from build123d import *

# Parameters (mm, degrees)
SKETCH1_W               = 167
SKETCH1_H               = 140.66
BOSS_EXTRUDE1_DEPTH     = 2
BOSS_EXTRUDE1_DRAFT     = -45
CUT_EXTRUDE1_REACH      = 220.353
SKETCH2_W               = 167
SKETCH2_H               = 140.66
SKETCH2_W_2             = 165
SKETCH2_H_2             = 138.66
BOSS_EXTRUDE2_START     = 120
BOSS_EXTRUDE2_DEPTH     = 22
CUT_EXTRUDE2_REACH      = 211.584
SKETCH4_W               = 20
SKETCH4_H               = 20
CUT_EXTRUDE3_DEPTH      = 218.119588246
CUT_EXTRUDE3_DEPTH_BACK = 218.119588246
SKETCH5_W               = 9
SKETCH5_H               = 9
CUT_EXTRUDE4_REACH      = 219.12
SKETCH6_W               = 59.5
SKETCH6_H               = 89
SKETCH7_W               = 35
SKETCH7_H               = 51
CUT_EXTRUDE5_DEPTH      = 2
BOSS_EXTRUDE4_START     = -2
SKETCH11_W              = 39
SKETCH11_H              = 55
BOSS_EXTRUDE4_DEPTH     = 1
CUT_EXTRUDE6_DEPTH      = 218.119588246
CUT_EXTRUDE6_DEPTH_BACK = 218.119588246
SKETCH12_W              = 9
SKETCH12_H              = 9


with BuildPart() as part:
    # Sketch1 → Boss-Extrude1 (with draft: the straight prism first)
    with BuildSketch(Plane(origin=(0, 0, 0), x_dir=(1, 0, 0), z_dir=(0, 1, 0))):
        with Locations((83.5, 70.33)):
            Rectangle(SKETCH1_W, SKETCH1_H)
    extrude(amount=-BOSS_EXTRUDE1_DEPTH)
    # Boss-Extrude1: the draft: its side faces are tilted about the plane it starts from
    boss_extrude1_sides = [part.faces().sort_by_distance(p)[0] for p in [
        (83.5, -1, 0),
        (167, -1, -70.33),
        (83.5, -1, -140.66),
        (0, -1, -70.33),
    ]]
    draft(boss_extrude1_sides, Plane(origin=(0, 0, 0), x_dir=(1, 0, 0), z_dir=(0, 1, 0)), BOSS_EXTRUDE1_DRAFT)

    # Sketch2 → Cut-Extrude1 (cut, up to next)
    with BuildSketch(Plane.XZ.offset(2), mode=Mode.PRIVATE) as cut_extrude1_sk1:
        with Locations((83.5, -70.33)):
            Rectangle(SKETCH2_W, SKETCH2_H)
        with Locations((83.5, -70.33)):
            Rectangle(SKETCH2_W_2, SKETCH2_H_2, mode=Mode.SUBTRACT)
    cut_extrude1_tool1 = extrude(cut_extrude1_sk1.sketch, amount=-CUT_EXTRUDE1_REACH, mode=Mode.PRIVATE) & part.part
    add(cut_extrude1_tool1.solids().sort_by_distance((83.5, -2, -140.441656))[0], mode=Mode.SUBTRACT)

    # Sketch3 → Boss-Extrude2 (add)
    with BuildSketch(Plane(origin=(0, 0, 0), x_dir=(0, 0, -1), z_dir=(1, 0, 0)).offset(BOSS_EXTRUDE2_START)):
        Polygon((76.33, 0), (84.33, 8.94427191), (103.33, 0), align=None)
    extrude(amount=BOSS_EXTRUDE2_DEPTH)

    # Cut-Extrude2: up to this plane
    cut_extrude2_end = Plane(origin=(0, -2, 0), z_dir=(0, -1, 0))
    # Sketch4 → Cut-Extrude2 (cut, up to the surface)
    with BuildSketch(Plane(origin=(0, 39.818641072, -18.744671202), x_dir=(1, 0, 0), z_dir=(0, 0.9047619047619048, -0.42591770999996015)), mode=Mode.PRIVATE) as cut_extrude2_sk1:
        with Locations((131, 83.489047619)):
            Rectangle(SKETCH4_W, SKETCH4_H)
    cut_extrude2_tool1 = split(extrude(cut_extrude2_sk1.sketch, amount=-CUT_EXTRUDE2_REACH, mode=Mode.PRIVATE), bisect_by=cut_extrude2_end, keep=Keep.BOTH, mode=Mode.PRIVATE)
    add(cut_extrude2_tool1.solids().sort_by_distance((131, 4.259177, -94.282381))[0], mode=Mode.SUBTRACT)

    # Sketch5 → Cut-Extrude3 (cut, two sides: drawn at the far end of the back side and taken through both)
    with BuildSketch(Plane(origin=(0, 0, 0), x_dir=(1, 0, 0), z_dir=(0, 1, 0)).offset(-CUT_EXTRUDE3_DEPTH_BACK)):
        with Locations((92, 90.33)):
            Rectangle(SKETCH5_W, SKETCH5_H)
        with Locations((92, 52.33)):
            Rectangle(SKETCH5_W, SKETCH5_H)
        with Locations((70, 52.33)):
            Rectangle(SKETCH5_W, SKETCH5_H)
    extrude(amount=CUT_EXTRUDE3_DEPTH + CUT_EXTRUDE3_DEPTH_BACK, mode=Mode.SUBTRACT)

    # Sketch6 → Cut-Extrude4 (cut, up to next)
    with BuildSketch(Plane(origin=(0, 0, 0), x_dir=(1, 0, 0), z_dir=(0, 1, 0)), mode=Mode.PRIVATE) as cut_extrude4_sk1:
        with Locations((31.75, 79.33)):
            Rectangle(SKETCH6_W, SKETCH6_H)
    cut_extrude4_tool1 = extrude(cut_extrude4_sk1.sketch, amount=-CUT_EXTRUDE4_REACH, mode=Mode.PRIVATE) & part.part
    add(cut_extrude4_tool1.solids().sort_by_distance((31.75, 0, -79.33))[0], mode=Mode.SUBTRACT)

    # Sketch7 → Cut-Extrude5 (cut)
    with BuildSketch(Plane(origin=(0, 0, 0), x_dir=(1, 0, 0), z_dir=(0, 1, 0))):
        with Locations((81, 71.33)):
            Rectangle(SKETCH7_W, SKETCH7_H)
    extrude(amount=-CUT_EXTRUDE5_DEPTH, mode=Mode.SUBTRACT)

    # Sketch11 → Boss-Extrude4 (add)
    with BuildSketch(Plane(origin=(0, 0, 0), x_dir=(1, 0, 0), z_dir=(0, 1, 0)).offset(BOSS_EXTRUDE4_START)):
        with Locations((81, 71.33)):
            Rectangle(SKETCH11_W, SKETCH11_H)
    extrude(amount=-BOSS_EXTRUDE4_DEPTH)

    # Sketch12 → Cut-Extrude6 (cut, two sides: drawn at the far end of the back side and taken through both)
    with BuildSketch(Plane(origin=(0, 0, 0), x_dir=(1, 0, 0), z_dir=(0, 1, 0)).offset(-CUT_EXTRUDE6_DEPTH_BACK)):
        with Locations((92, 52.33)):
            Rectangle(SKETCH12_W, SKETCH12_H)
        with Locations((70, 52.33)):
            Rectangle(SKETCH12_W, SKETCH12_H)
        with Locations((92, 90.33)):
            Rectangle(SKETCH12_W, SKETCH12_H)
    extrude(amount=CUT_EXTRUDE6_DEPTH + CUT_EXTRUDE6_DEPTH_BACK, mode=Mode.SUBTRACT)


solid = part.part
Design review of the part built by this model. Coordinates are the model's own, in mm. A direction names the side the tool comes from. Coordinates: 2 decimals unless noted, no trailing zeros. Order: outer loops, then holes, each group sorted by start corner. A loop starts at its lowest first (then second) coordinate and runs counter-clockwise, first axis right, second up. Notation, with made-up numbers: (37, 47.5) -> (81, 47.5) arc R3 ccw to (81, 51.5) -> close; hole circle Ø2 at (77.25, 22.25). An arc over 180 degrees is marked (long way). Use one line per item in the form item = value. Start each with the question number.
(1) Add section C-C on z = -64. State the section outline as (x, y) points.
(2) Add section B-B on x = 47. State the section outline as (y, z) points.
(3) For faces 5 (the flat face through (81, -2, -72)), 6 (the flat face through (130.95, 8.8, -84.64)), list the 3-axis set-ups (+Z, -Z, +X, -X, +Y, -Y) from which the entire face can be reached by the end or side of a thin tool; tool diameter is ignored.
(4) Add section A-A on z = -116. State the section outline as (x, y) points, plus the area to 3 significant figures.
(5) For probe 1 along X at (y, z) = (6.75, -85); probe 2 along X at (y, z) = (-0.5, -81.5); probe 3 along X at (y, z) = (-1.75, -80), list the stretches that pass through material, from the lowest coordinate up.
(6) Insertion check: pin 1 (17.5 mm diameter, centred on x = 84, z = -82, fed in from +Y); pin 2 (2 mm diameter, centred on y = 5, z = -77, fed in from +X); pin 3 (1.1 mm diameter, centred on x = 85, y = -2.5, fed in from +Z); pin 4 (8 mm diameter, centred on x = 39.5, z = -125, fed in from -Y). Each pin has a flat end and moves straight along its axis. Give the tip position at first contact, or say it passes through.
(7) The part is to be moulded in two halves that separate along X. For faces 1 (the flat face through (81, -3, -72)), 2 (the flat face through (142, 4, -87)), 3 (the flat face through (120, 4, -87)), 4 (the flat face through (130.86, 3.333, -82.794)), say which applies: +X half, -X half, draft (parallel to the pull), parting line (faces both ways), or undercut.
(8) Add section D-D on y = 3. State the section outline as (x, z) points, plus the area to 3 significant figures.
Answer block:
q1.outline = (1, -1) -> (2, -2) -> (2, 0) -> (1, 0) -> close; (61.5, -3) -> (100.5, -3) -> (100.5, -2) -> (165, -2) -> (166, -1) -> (166, 0) -> (98.5, 0) -> (98.5, -2) -> (63.5, -2) -> (63.5, 0) -> (61.5, 0) -> close
q2.outline = (-2, -138.66) -> (-1, -139.66) -> (0, -139.66) -> (0, -123.83) -> (-2, -123.83) -> close; (-2, -34.83) -> (0, -34.83) -> (0, -1) -> (-1, -1) -> (-2, -2) -> close
q3.face_5 = +Y
q3.face_6 = -Z, +X, -X, +Y
q4.outline = (1, -1) -> (2, -2) -> (2, 0) -> (1, 0) -> close; (61.5, -2) -> (165, -2) -> (166, -1) -> (166, 0) -> (61.5, 0) -> close
q4.area = 210 mm²
q5.probe_1 = 120 to 121, 141 to 142
q5.probe_2 = 1 to 2, 61.5 to 63.5, 98.5 to 121, 141 to 166
q5.probe_3 = 1.75 to 2, 61.5 to 63.5, 98.5 to 165.25
q6.pin_1 = -2
q6.pin_2 = through
q6.pin_3 = -1.95
q6.pin_4 = -2
q7.face_1 = draft
q7.face_2 = +X half
q7.face_3 = -X half
q7.face_4 = undercut
q8.outline = (120, -96.96) -> (121, -96.96) -> (121, -82.64) -> (141, -82.64) -> (141, -96.96) -> (142, -96.96) -> (142, -79.01) -> (120, -79.01) -> close
q8.area = 108 mm²
